CAD build for the part. Positions are in the model's coordinates, mm. A direction names the side the tool comes from. Coordinates: 2 decimals unless noted, no trailing zeros. Loops run counter-clockwise (first coordinate to the right, second up) from the corner with the lowest first, then second, coordinate; pieces in that order, holes last. Notation, with made-up numbers: (23, 2.5) -> (69, 2.5) arc R25 cw to (69, 33.5) -> close; hole circle Ø7 at (6.25, 23.25). An arc over 180 degrees is marked (long way). Write each question's results on one line, items separated by ' | '.
from build123d import *

# Parameters (mm, degrees)
F0_W     = 59
F0_H     = 41
F1_DEPTH = 21
F2_R     = 10
F3_DEPTH = 8
F4_R     = 6
F5_DEPTH = 1


with BuildPart() as f1:
    # F0 (on Top) → F1 (new body)
    with BuildSketch(Plane.XY):
        Rectangle(F0_W, F0_H)
    extrude(amount=F1_DEPTH)

    # F2 (on face) → F3 (join)
    with BuildSketch(Plane.XY.offset(21)):
        with Locations((9.5, 0)):
            Circle(F2_R)
    extrude(amount=F3_DEPTH)

    # F4 (on face) → F5 (join)
    with BuildSketch(Plane(origin=(0, 20.5, 0), x_dir=(-1, 0, 0), z_dir=(0, 1, 0))):
        with Locations((17.5, 10.5)):
            Circle(F4_R)
    extrude(amount=F5_DEPTH)


solid = f1.part
1) Pin check, flat tips, straight feed: pin 1 (2 mm diameter, centred on x = -5.5, y = 7.5, fed in from -Z); pin 2 (4 mm diameter, centred on y = 1.5, z = 23.5, fed in from +X); pin 3 (2 mm diameter, centred on x = 15.5, z = 8, fed in from +Y); pin 4 (3 mm diameter, centred on y = -6.5, z = 23.5, fed in from +X). Stop position of each tip, or through.
Outcome:
pin 1: stops at z = 0 | pin 2: stops at x = 19.5 | pin 3: stops at y = 20.5 | pin 4: stops at x = 18.16
2) Slice it at B-B (z = 10.5). Write the cut outline in (x, y), then the cut area to 3 significant figures.
Outcome:
outline: (-29.5, -20.5) -> (29.5, -20.5) -> (29.5, 20.5) -> (-11.5, 20.5) -> (-11.5, 21.5) -> (-23.5, 21.5) -> (-23.5, 20.5) -> (-29.5, 20.5) -> close | area: 2,430 mm^2
3) Slice it at C-C (x = -5). Write the cut outline in (y, z).
Outcome:
outline: (-20.5, 0) -> (20.5, 0) -> (20.5, 21) -> (-20.5, 21) -> close
4) Which spindle directions (+Z, -Z, +X, -X, +Y, -Y) get a long thin tool onto all of the face, cutting with end or side? Do faces 1 (the flat face through (29.5, 0, 10)), 2 (the cylindrical face through (-23.04, 20.99, 8.2)), 3 (the cylindrical face through (-0.49, 0.44, 24.94)). Say none if no direction does.
Outcome:
face 1: +Z, -Z, +X, +Y, -Y | face 2: +Y | face 3: +Z
5) Drill centre lines: L1, parallel to Y at x = 16, z = 2.5; L2, parallel to Z at x = -1, y = 13.5; L3, parallel to Y at x = 5.5, z = 27.25. Where is each one in solid material? Low to high. Write a range as from..to.
Outcome:
L1: y = -20.5..20.5 | L2: z = 0..21 | L3: y = -9.17..9.17
6) Slice it at A-A (y = 8). Write the cut outline in (x, z), then the cut area to 4 significant figures.
Outcome:
outline: (-29.5, 0) -> (29.5, 0) -> (29.5, 21) -> (15.5, 21) -> (15.5, 29) -> (3.5, 29) -> (3.5, 21) -> (-29.5, 21) -> close | area: 1,335 mm^2
7) Slice it at D-D (y = -14). Write the cut outline in (x, z).
Outcome:
outline: (-29.5, 0) -> (29.5, 0) -> (29.5, 21) -> (-29.5, 21) -> close
